The listing builds one solid part. Answer for the finished solid, in the listing's coordinates (mm). Face numbers are marked on the shaded views. Coordinates: 2 decimals unless noted, no trailing zeros. Answer as CSV lines item,"result".
```python
from build123d import *

# Parameters (mm, degrees)
F0_W      = 120
F0_H      = 150
F1_DEPTH  = 30
F1_FACE_W = 120
F1_FACE_H = 150
F3_W      = 80
F3_H      = 110
F5_R      = 30


with BuildPart() as f1:
    # F0 (on Top) → F1 (new body)
    with BuildSketch(Plane.XY):
        with Locations((60, 75)):
            Rectangle(F0_W, F0_H)
    extrude(amount=F1_DEPTH)

    # F1_face (on face) → F4 section 0
    with BuildSketch(Plane(origin=(60, 75, 30), x_dir=(1, 0, 0), z_dir=(0, 0, 1))):
        Rectangle(F1_FACE_W, F1_FACE_H)
    # F3 (on offset) → F4 section 1
    with BuildSketch(Plane.XY.offset(25)):
        with Locations((60, 75)):
            Rectangle(F3_W, F3_H)
    loft(mode=Mode.SUBTRACT)

    # F5
    f5_edges = [f1.edges().sort_by_distance(p)[0] for p in [
        (20, 75, 25),
        (60, 20, 25),
        (100, 75, 25),
        (60, 130, 25),
    ]]
    fillet(f5_edges, radius=F5_R)


solid = f1.part
```
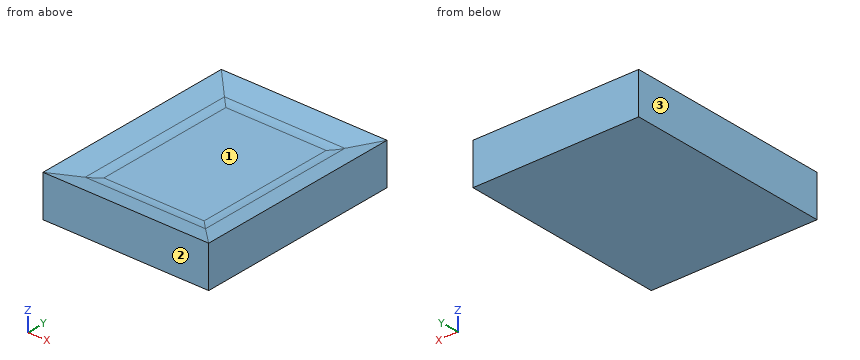
Q1. Flat-ended cylindrical pins translate along their axes: pin 1 Ø10 at (x, y) = (31, 62) entering from +Z; pin 2 Ø10 at (x, y) = (26.5, 61.5) entering from +Z. Find the tip coordinate at first contact, or state that the pin passes through.
Output:
pin 1,"z = 25"
pin 2,"z = 25.08"
Q2. Straight lines are drawn through the part: line 1 (Z direction, x = 38, y = 122); line 2 (Z direction, x = 6, y = 88.5). For each, find the intervals that lie inside material, in ascending order.
Output:
line 1,"0 to 25"
line 2,"0 to 28.5"
Q3. The mould has two halves that part along X. Classify the marked faces 1, 2 and 3: pulls with the +X half, pulls with the -X half, needs draft (parallel to the pull), parting line crosses it, or undercut.
Output:
face 1,"undercut"
face 2,"needs draft"
face 3,"pulls with the -X half"
